Build history of the part. All positions in model axes, mm. A direction names the side the tool comes from. Give positions to 0.01 mm unless a question says otherwise; leave off trailing zeros. Order: outer loops, then holes, each group sorted by start corner. A loop starts at its lowest first (then second) coordinate and runs counter-clockwise, first axis right, second up. Notation, with made-up numbers: M 20,30 L 61,30 A21 cw 61,37 Z; hole C 14.25,9.5 d1. An arc over 180 degrees is marked long. One line per item, written item: value. Start each with the question number.
from build123d import *

# Parameters (mm, degrees)
DODANIE_WYCI_GNI_CIE2_DEPTH = 20
SZKIC28_W                   = 16.8
SZKIC28_H                   = 16.8
WYTNIJ_WYCI_GNI_CIE1_DEPTH  = 20
SZKIC29_W                   = 16.8
SZKIC29_H                   = 16.8
WYTNIJ_WYCI_GNI_CIE2_DEPTH  = 20


with BuildPart() as part:
    # Szkic1 → Dodanie-wyciągnięcie2 (new body)
    with BuildSketch(Plane.XY):
        with BuildLine():
            Line((40, 40), (348.019609728, 40))
            ThreePointArc((348.019609728, 40), (402.791865479, 29.642400438), (450, 0))
            Line((450, 0), (417.280680948, 0))
            ThreePointArc((417.280680948, 0), (382.503671889, 22.185117958), (342, 30))
            Line((342, 30), (116.308192204, 30))
            Line((116.308192204, 30), (90, 30))
            ThreePointArc((90, 30), (68.786796564, 21.213203436), (60, 0))
            Line((60, 0), (0, 0))
            ThreePointArc((0, 0), (11.715728753, 28.284271247), (40, 40))
        make_face()
    extrude(amount=DODANIE_WYCI_GNI_CIE2_DEPTH)

    # Szkic28 → Wytnij-wyciągnięcie1 (cut)
    with BuildSketch(Plane(origin=(0, 30, 0), x_dir=(1, 0, 0), z_dir=(0, 1, 0))):
        with Locations((26.6, -10)):
            Rectangle(SZKIC28_W, SZKIC28_H)
    extrude(amount=WYTNIJ_WYCI_GNI_CIE1_DEPTH, mode=Mode.SUBTRACT)

    # Szkic29 → Wytnij-wyciągnięcie2 (cut)
    with BuildSketch(Plane(origin=(0, 10, 0), x_dir=(1, 0, 0), z_dir=(0, 1, 0))):
        with Locations((428.1, -10)):
            Rectangle(SZKIC29_W, SZKIC29_H)
    extrude(amount=WYTNIJ_WYCI_GNI_CIE2_DEPTH, mode=Mode.SUBTRACT)

    # Szkic32 → Pog_bienie walcowe pod M6 wkr_t z _bem s (revolve, cut)
    with BuildSketch(Plane(origin=(428.1, 10, 10), x_dir=(0, 0, 1), z_dir=(1, 0, 0))):
        Polygon((0, 0), (0, 26.922753981), (3.2, 25), (3.2, 4), (7.2735, 4), (7.2735, 0.025), (7.2985, 0), align=None)
    revolve(axis=Axis((428.1, 16.35, 10), (0, -1, 0)), mode=Mode.SUBTRACT)

    # Szkic34 → Pog_bienie walcowe pod M6 wkr_t z _b 2 (revolve, cut)
    with BuildSketch(Plane(origin=(26.6, 30, 10), x_dir=(0, 0, 1), z_dir=(1, 0, 0))):
        Polygon((0, 0), (0, 41.922753981), (3.2, 40), (3.2, 4), (7.2735, 4), (7.2735, 0.025), (7.2985, 0), align=None)
    revolve(axis=Axis((26.6, 36.35, 10), (0, -1, 0)), mode=Mode.SUBTRACT)


solid = part.part
1) Drop flat-ended pins along their axis: P1, Ø5, axis at y = 36, z = 10.5, coming from the -X side; P2, Ø3, axis at x = 288, z = 12, coming from the -Y side; P3, Ø12, axis at x = 351.5, z = 16.5, coming from the -Y side. Give the stop position or say it passes through.
2) Drill centre lines: line 1 (Z direction, x = 26, y = 13); line 2 (Z direction, x = 428, y = 7); line 3 (X direction, y = 1.6, z = 10). Where is each one in solid material? Low to high.
3) Slice it at C-C (x = 333). List the corners of the cut face in (y, z), plus the area to 3 significant figures.
4) Pull direction X, two halves, no side cores. Call faces 1 (the cylindrical face through (69.021, 21.445, 9.86)), 2 (the cylindrical face through (390.26, 33.93, 9.86)), 3 (the flat face through (192, 40, 10)): pulls with the +X half, pulls with the -X half, needs draft (parallel to the pull), parting line crosses it, or undercut.
5) Slice it at B-B (z = 10). State how many separate pieces and enclosed holes the cut face has, plus the area to 3 significant figures.
6) Tool access for faces 4 (the cylindrical face through (383.04, 21.97, 9.86)), 5 (the cylindrical face through (6.984, 22.581, 9.86)), 6 (the cylindrical face through (20.467, 28.015, 13.91)): list every direction of +Z, -Z, +X, -X, +Y, -Y with a clear straight run to the whole face (end or side of a thin tool).
7) Slice it at A-A (y = 16.5). List the corners of the cut face in (x, z).
Results list:
1. P1: stops at x = 18.14
1. P2: stops at y = 30
1. P3: stops at y = 28.87
2. line 1: z = 0 to 6.86, 13.14 to 20
2. line 2: z = 0 to 2.73, 17.27 to 20
2. line 3: x = 0.03 to 23.4, 29.8 to 60.04, 415.55 to 424.9, 431.3 to 448.25
3. outline: M 30,0 L 40,0 L 40,20 L 30,20 Z
3. area: 200 mm²
4. face 1: undercut
4. face 2: pulls with the +X half
4. face 3: needs draft
5. separate pieces: 3
5. enclosed holes: 0
5. area: 6,000 mm²
6. face 4: +Z, -Z, -Y
6. face 5: +Z, -Z, -X, +Y
6. face 6: +Y
7. outline: M 3.56,0 L 64.95,0 L 64.95,20 L 3.56,20 Z; M 394.58,0 L 428.63,0 L 428.63,1.6 L 419.7,1.6 L 419.7,18.4 L 428.63,18.4 L 428.63,20 L 394.58,20 Z; hole C 26.6,10 d6.4
